Autodesk Inventor part; units mm, degrees
ref_plane "YZ Plane" through (0, 0, 0) normal (1, 0, 0) x (0, 1, 0)
ref_plane "XZ Plane" through (0, 0, 0) normal (0, 1, 0) x (-1, 0, 0)
ref_plane "XY Plane" through (0, 0, 0) normal (0, 0, 1) x (1, 0, 0)
sketch "Sketch5" plane through (0, 0, 0) normal (0, 1, 0) x (-1, 0, 0)
  line L0 (0, 0) -> (-20, 0)
  line L1 (-20, 0) -> (-20, -20)
  line L2 (-20, -20) -> (0, -20)
  line L3 (0, -20) -> (0, 0)
  dimension "d13" = 20
extrude "Plate2" add sketch "Sketch5" along normal blind 0.5
sketch "Sketch6" plane through (0, 0.5, 0) normal (0, 1, 0) x (1, 0, 0)
  circle A0 centre (10, 10) radius 6
  line L0 (0, 20) -> (20, 20) construction
  line L1 (20, 20) -> (20, 0) construction
  line L2 (10, 10) -> (10, 4) construction
  point P0 (0, 0)
  dimension "d15" = 12
  dimension "d16" = 10
  dimension "d17" = 10
extrude "Extrusion2" cut sketch "Sketch6" against normal blind 0.5
ref_plane "Work Plane2" through (10, 0.5, -10) normal (0, 0, 1) x (1, 0, 0)
sketch "Sketch7" plane through (10, 0.5, -10) normal (0, 0, 1) x (1, 0, 0)
  line L0 (6, 0) -> (-6, 0)
  arc A0 (-2.2412, -2.6319) -> (-6, 0) centre (-6, -4) ccw
  line L1 (0, 0) -> (0, -5) construction
  line L2 (-2.2412, -2.6319) -> (-1.3793, -5)
  line L3 (-1.3793, -5) -> (-1.8492, -5.171)
  line L4 (-1.8492, -5.171) -> (-2.7111, -2.8029)
  line L5 (-6, 0) -> (-6, -0.5)
  arc A1 (-2.7111, -2.8029) -> (-6, -0.5) centre (-6, -4) ccw
  point P0 (-10, -0.5)
  dimension "d20" = 5
  dimension "d21" = 20
  dimension "d22" = 4
  dimension "d23" = 0.5
revolve "Revolution2" add sketch "Sketch7" angle 360 about axis through (10, 0.5, -10) along (0, -1, 0)
equation "\"d18\" = Thickness"
equation "\"d23\" = Thickness"
equation "\"d14\" = Thickness"
equation "\"BendRadius\" = Thickness"
equation "\"BendReliefWidth\" = Thickness"
equation "\"BendReliefDepth\" = 0.5 * Thickness"
equation "\"CornerReliefSize\" = 4 * Thickness"
equation "\"MinimumRemnant\" = 2 * Thickness"
equation "\"TransitionRadius\" = BendRadius"
equation "\"JacobiRadiusSize\" = BendRadius"
equation "\"GapSize\" = Thickness"
properties part number "CE-4.1.1"
Part model, mm, in its own coordinate system. Round coordinates to 2 decimals unless told otherwise and drop trailing zeros. Write each loop counter-clockwise with the first axis right and the second up, starting at its lowest first coordinate (ties: lowest second). Pieces come first, ordered by that corner, then holes. Notation, with made-up numbers: M -22.5,52.25 L 1.5,52.25 A10 ccw 1.5,63.25 Z; hole C -11.5,63 d10. An arc over 180 degrees is marked long. Return JSON: item names as keys, results as strings. Group by question number.
(1) Saw through at D-D on z = -18. Write the cut outline in (x, y), then the cut area to 3 significant figures.
(2) Drill centre lines: probe 1 along Y at (x, z) = (16.5, -10); probe 2 along X at (y, z) = (-3.85, -9.25); probe 3 along X at (y, z) = (-1.05, -8.5). Where is each one in solid material? Low to high.
(3) Two-plate mould, pull along Z, no slides. Class faces 1 (the face through (11.473, -4.26, -8.649)), 2 (the face through (6, 0.5, -5)), 3 (the face through (8.45, -3.826, -9.512)): +Z half, -Z half, draft (parallel to the pull), parting line (faces both ways), or undercut.
(4) Pin check, flat tips, straight feed: pin 1 Ø4 at (x, z) = (16.5, -6) entering from -Y; pin 2 Ø5 at (x, z) = (12, -3.5) entering from -Y. Stop position of each tip, or through.
(5) Saw through at B-B on z = -10. Write the cut outline in (x, y).
(6) Saw through at C-C on y = -3.5. Write the cut outline in (x, z), then the cut area to 3 significant figures.
(7) Saw through at A-A on x = 10. Write the cut outline in (y, z), then the cut area to 3 significant figures.
Returned:
{
 "1": {"outline": "M 0,0 L 20,0 L 20,0.5 L 0,0.5 Z", "area": "10.0 mm²"},
 "2": {"probe 1": "0 to 0.5", "probe 2": "7.99 to 8.57, 11.43 to 12.01", "probe 3": "6.84 to 7.59, 12.41 to 13.16"},
 "3": {"face 1": "parting line", "face 2": "draft", "face 3": "undercut"},
 "4": {"pin 1": "y = -0.02", "pin 2": "y = -0.44"},
 "5": {"outline": "M 0,0 L 4,0 A3.5 cw 7.29,-2.3 L 8.15,-4.67 L 8.62,-4.5 L 7.76,-2.13 A4 ccw 4,0.5 L 0,0.5 Z; M 11.38,-4.5 L 11.85,-4.67 L 12.71,-2.3 A3.5 cw 16,0 L 20,0 L 20,0.5 L 16,0.5 A4 ccw 12.24,-2.13 Z"},
 "6": {"outline": "C 10,-10 d4.55; hole C 10,-10 d3.49", "area": "6.72 mm²"},
 "7": {"outline": "M -4.67,-11.85 L -2.3,-12.71 A3.5 cw 0,-16 L 0,-20 L 0.5,-20 L 0.5,-16 A4 ccw -2.13,-12.24 L -4.5,-11.38 Z; M -4.67,-8.15 L -4.5,-8.62 L -2.13,-7.76 A4 ccw 0.5,-4 L 0.5,0 L 0,0 L 0,-4 A3.5 cw -2.3,-7.29 Z", "area": "11.1 mm²"}
}
